Check sheet for the drawn part. Datum: minimum x, y, z corner. Units: mm. A direction names the side the tool comes from. Round coordinates to 2 decimals unless told otherwise and drop trailing zeros. Loops run counter-clockwise (first coordinate to the right, second up) from the corner with the lowest first, then second, coordinate; pieces in that order, holes last.
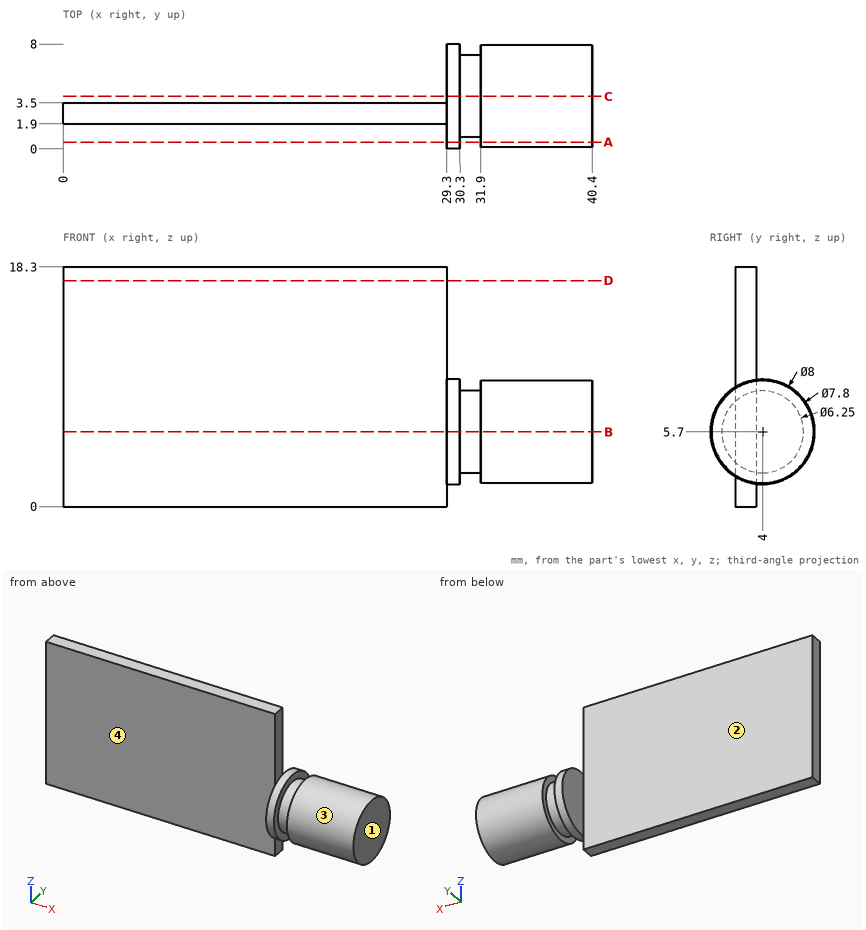
1) Scan lines: line 1 along X through (y, z) = (1.5, 4.25); line 2 along Y through (x, z) = (16, 7.25); line 3 along Z through (x, y) = (34, 4.25). Record each from-to range of solid material in increasing order.
Report:
line 1: x = 29.3 to 40.4
line 2: y = 1.9 to 3.5
line 3: z = 1.81 to 9.59
2) Sectioned sample at A-A, the plane y = 0.5. Record the cut outline in (x, z).
Report:
outline: (29.3, 3.76) - (30.3, 3.76) - (30.3, 7.64) - (29.3, 7.64) - close; (31.9, 3.98) - (40.4, 3.98) - (40.4, 7.42) - (31.9, 7.42) - close
3) Gauge pin test, flat ends, axial feed: pin 1 (3 mm diameter, centred on y = 6, z = 3.5, fed in from -X); pin 2 (5.5 mm diameter, centred on x = 9.5, z = 9, fed in from -Y); pin 3 (9 mm diameter, centred on x = 8, z = 7.5, fed in from +Y). Record the tip position at first contact, or that the pin passes through.
Report:
pin 1: stops at x = 29.3
pin 2: stops at y = 1.9
pin 3: stops at y = 3.5
4) Sectioned sample at C-C, the plane y = 4. Record the cut outline in (x, z) (3 decimals).
Report:
outline: (29.3, 1.7) - (30.3, 1.7) - (30.3, 2.575) - (31.9, 2.575) - (31.9, 1.8) - (40.4, 1.8) - (40.4, 9.6) - (31.9, 9.6) - (31.9, 8.825) - (30.3, 8.825) - (30.3, 9.7) - (29.3, 9.7) - close
5) Sectioned sample at D-D, the plane z = 17.25. Record the cut outline in (x, y), then the cut area to 3 significant figures.
Report:
outline: (0, 1.9) - (29.3, 1.9) - (29.3, 3.5) - (0, 3.5) - close
area: 46.9 mm2
6) Access from +Z, -Z, +X, -X, +Y, -Y to the whole of each face (thin tool, end or side, straight path). Record for the marked faces 1, 2, 3 and 4.
Report:
face 1: +Z, -Z, +X, +Y, -Y
face 2: +Z, -Z, -X, +Y
face 3: +X
face 4: +Z, -Z, -X, -Y
7) Sectioned sample at B-B, the plane z = 5.7. Record the cut outline in (x, y) (3 decimals), then the cut area to 3 significant figures.
Report:
outline: (0, 1.9) - (29.3, 1.9) - (29.3, 0) - (30.3, 0) - (30.3, 0.875) - (31.9, 0.875) - (31.9, 0.1) - (40.4, 0.1) - (40.4, 7.9) - (31.9, 7.9) - (31.9, 7.125) - (30.3, 7.125) - (30.3, 8) - (29.3, 8) - (29.3, 3.5) - (0, 3.5) - close
area: 131 mm2
